Could you check a few things on this drawing? It's one solid part, dimensions in mm from its lowest x, y, z. Give positions to 0.01 mm unless a question says otherwise; leave off trailing zeros. Loops run counter-clockwise (first coordinate to the right, second up) from the corner with the lowest first, then second, coordinate; pieces in that order, holes last. Notation, with made-up numbers: M -39.75,-22.75 L 14.25,-22.75 A33 ccw 14.25,14.25 Z; hole C -5.5,-35 d7. An arc over 180 degrees is marked long. Answer in a Markdown table with one row per item. Add a question column.
1. I need wall thicknesses on line 1 along X through (y, z) = (14, 1.75); line 2 along X through (y, z) = (16.5, 2.5); line 3 along Y through (x, z) = (17.5, 6.75) (1 decimal). Which ranges of each line are inside material? Lowest first, please. Write a range as from..to.
2. I'm going to push a flat-ended pin straight in: pin 1 Ø1.5 at (x, z) = (7.5, 3) entering from -Y (1 decimal). Where does the tip first touch, or does it pass through?
3. Thinking about a two-plate mould opening in X: for the marked faces 1, 2, 3 and 4, which applies, released by +X, released by -X, zero draft, split by the parting line, or undercut?
4. If we section it at A-A on z = 2.25: List the corners of the cut face in (x, y) for me (1 decimal), then the cut area to 3 significant figures.
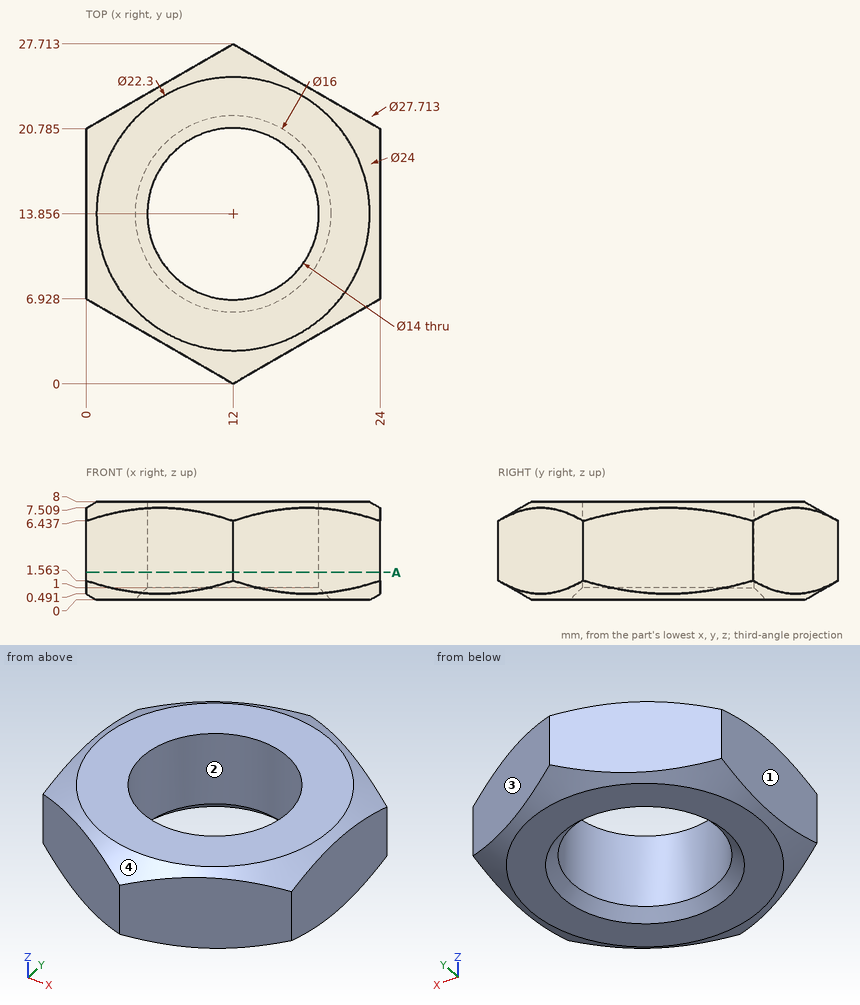
Results:
| question | item | result |
|---|---|---|
| 1 | line 1 | 0..5, 19..24 |
| 1 | line 2 | 0..5.52, 18.48..24 |
| 1 | line 3 | 3.2..9.5, 18.2..24.5 |
| 2 | pin 1 | y = 2.2 |
| 3 | face 1 | released by -X |
| 3 | face 2 | undercut |
| 3 | face 3 | released by +X |
| 3 | face 4 | split by the parting line |
| 4 | outline | M 0,6.9 L 12,0 L 24,6.9 L 24,20.8 L 12,27.7 L 0,20.8 Z; hole C 12,13.9 d14 |
| 4 | area | 345 mm2 |
